Check sheet for the drawn part. Datum: minimum x, y, z corner. Units: mm. A direction names the side the tool comes from. Coordinates: 2 decimals unless noted, no trailing zeros. Loops run counter-clockwise (first coordinate to the right, second up) from the corner with the lowest first, then second, coordinate; pieces in that order, holes last.
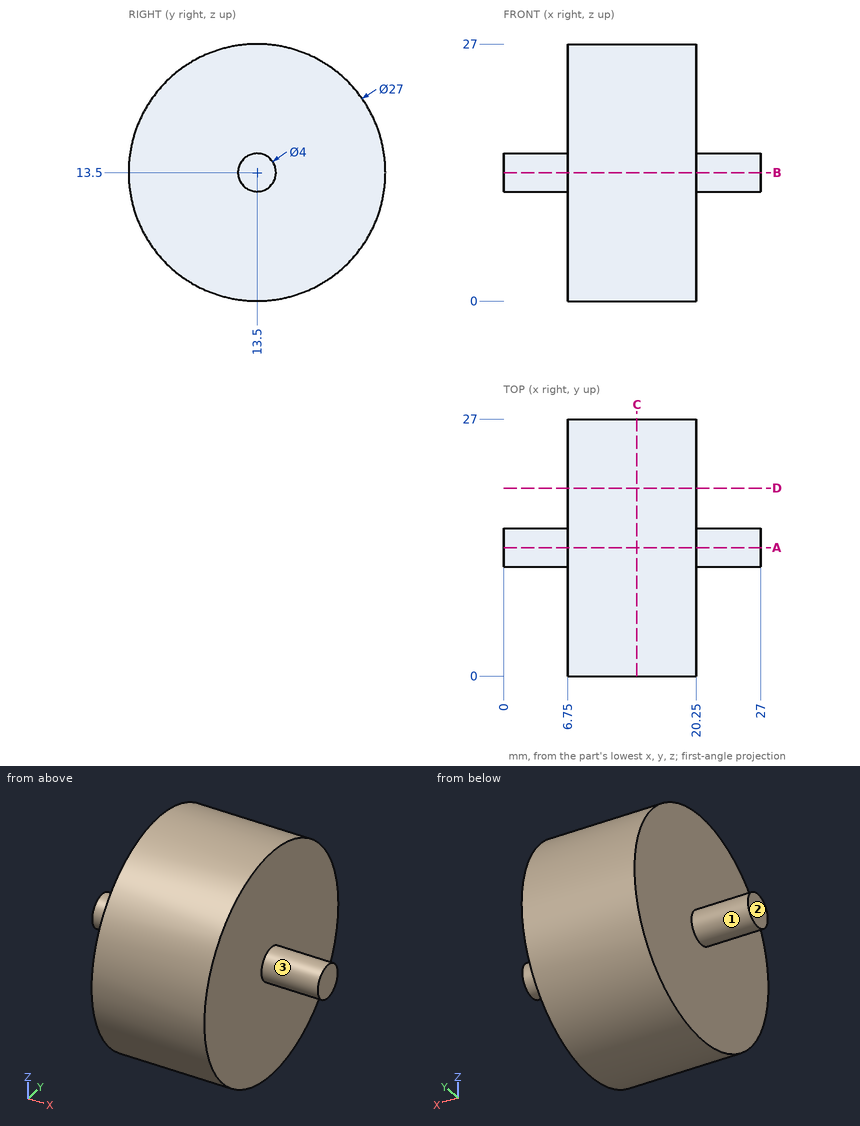
(1) Access from +Z, -Z, +X, -X, +Y, -Y to the whole of each face (thin tool, end or side, straight path). Record for the marked faces 1, 2 and 3.
Findings:
face 1: -X
face 2: +Z, -Z, -X, +Y, -Y
face 3: +X
(2) Sectioned sample at A-A on y = 13.5. Record the cut outline in (x, z), and give its area (4 significant figures).
Findings:
outline: (0, 11.5) - (6.75, 11.5) - (6.75, 0) - (20.25, 0) - (20.25, 11.5) - (27, 11.5) - (27, 15.5) - (20.25, 15.5) - (20.25, 27) - (6.75, 27) - (6.75, 15.5) - (0, 15.5) - close
area: 418.5 mm2
(3) Scan lines: L1, parallel to X at y = 1.75, z = 12.25; L2, parallel to Z at x = 1.5, y = 12.25; L3, parallel to Z at x = 15.5, y = 22. Record each from-to range of solid material in increasing order.
Findings:
L1: x = 6.75 to 20.25
L2: z = 11.94 to 15.06
L3: z = 3.01 to 23.99
(4) Gauge pin test, flat ends, axial feed: pin 1 Ø1.5 at (x, y) = (12, 9.5) entering from -Z; pin 2 Ø2 at (y, z) = (21.5, 15) entering from +X; pin 3 Ø4 at (x, y) = (20.5, 7.5) entering from +Z; pin 4 Ø10 at (y, z) = (15, 9) entering from -X. Record the tip position at first contact, or that the pin passes through.
Findings:
pin 1: stops at z = 0.4
pin 2: stops at x = 20.25
pin 3: stops at z = 26.39
pin 4: stops at x = 0
(5) Sectioned sample at D-D on y = 19.75. Record the cut outline in (x, z).
Findings:
outline: (6.75, 1.53) - (20.25, 1.53) - (20.25, 25.47) - (6.75, 25.47) - close
(6) Sectioned sample at C-C on x = 14. Record the cut outline in (y, z).
Findings:
outline: circle Ø27 at (13.5, 13.5)
